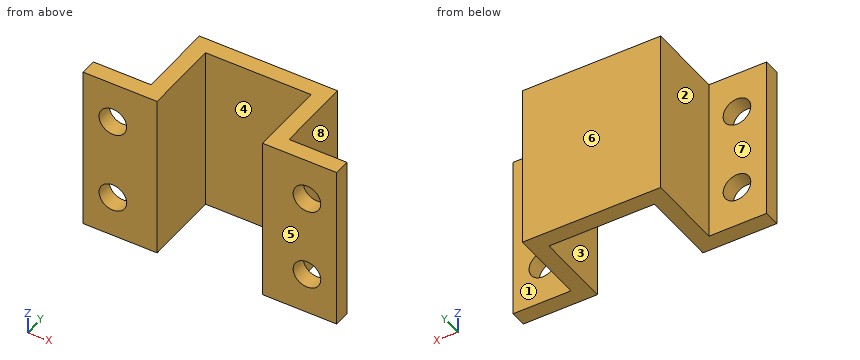
```python
from build123d import *

# Parameters (mm, degrees)
SKETCH1_W             = 9.1
SKETCH1_H             = 20.4
SKETCH1_R             = 1.7
BOSS_EXTRUDE1_DEPTH   = 2
BOSS_EXTRUDE1_2_DEPTH = 2
SKETCH2_W             = 2
SKETCH2_H             = 20.4
BOSS_EXTRUDE2_DEPTH   = 9.49
SKETCH3_W             = 17
SKETCH3_H             = 20.4
BOSS_EXTRUDE3_DEPTH   = 2


with BuildPart() as part:
    # Sketch1 → Boss-Extrude1 (new body)
    with BuildSketch(Plane(origin=(0, 0, 0), x_dir=(1, 0, 0), z_dir=(0, 1, 0))):
        with Locations((-11.05, 0)):
            Rectangle(SKETCH1_W, SKETCH1_H)
        with Locations(Location((-11.95, -5.1, 0), (0, 0, 270))):
            Circle(SKETCH1_R, mode=Mode.SUBTRACT)
        with Locations(Location((-11.95, 5.1, 0), (0, 0, 270))):
            Circle(SKETCH1_R, mode=Mode.SUBTRACT)
    extrude(amount=BOSS_EXTRUDE1_DEPTH)



with BuildPart() as body_2:
    # Sketch1 → Boss-Extrude1 2 (new body)
    with BuildSketch(Plane(origin=(0, 0, 0), x_dir=(1, 0, 0), z_dir=(0, 1, 0))):
        with Locations((11.05, 0)):
            Rectangle(SKETCH1_W, SKETCH1_H)
        with Locations(Location((11.95, -5.1, 0), (0, 0, 270))):
            Circle(SKETCH1_R, mode=Mode.SUBTRACT)
        with Locations(Location((11.95, 5.1, 0), (0, 0, 270))):
            Circle(SKETCH1_R, mode=Mode.SUBTRACT)
    extrude(amount=BOSS_EXTRUDE1_2_DEPTH)


with BuildPart() as part_1:
    add(part.part)

    add(body_2.part)  # Boss-Extrude2 merges body 2
    # Sketch2 → Boss-Extrude2 (add)
    with BuildSketch(Plane(origin=(0, 0, 0), x_dir=(1, 0, 0), z_dir=(0, 1, 0))):
        with Locations((-7.5, 0)):
            Rectangle(SKETCH2_W, SKETCH2_H)
        with Locations((7.5, 0)):
            Rectangle(SKETCH2_W, SKETCH2_H)
    extrude(amount=BOSS_EXTRUDE2_DEPTH)

    # Sketch3 → Boss-Extrude3 (add)
    with BuildSketch(Plane(origin=(0, 9.49, 0), x_dir=(1, 0, 0), z_dir=(0, 1, 0))):
        Rectangle(SKETCH3_W, SKETCH3_H)
    extrude(amount=BOSS_EXTRUDE3_DEPTH)


solid = part_1.part
```
Input: part model. Units: mm. Frame: model coordinates. Face numbers are marked on the shaded views. A direction names the side the tool comes from. Coordinates: 2 decimals unless noted, no trailing zeros. Loops run counter-clockwise (first coordinate to the right, second up) from the corner with the lowest first, then second, coordinate; pieces in that order, holes last. Notation, with made-up numbers: (-15, 37.5) - (26, 37.5) arc R13 cw to (26, 62.5) - close; hole circle Ø10 at (-30.5, 37). An arc over 180 degrees is marked (long way). Answer in a Markdown table with one row per item.
(1) Cut plane B-B on y = 8. Output: boundary loops of the cut face in (x, z), plus the area to 3 significant figures.
Model answer:
| item | result |
|---|---|
| outline | (-8.5, -10.2) - (-6.5, -10.2) - (-6.5, 10.2) - (-8.5, 10.2) - close; (6.5, -10.2) - (8.5, -10.2) - (8.5, 10.2) - (6.5, 10.2) - close |
| area | 81.6 mm² |
(2) Cut plane C-C on x = 11.95. Output: boundary loops of the cut face in (y, z), plus the area to 3 significant figures.
Model answer:
| item | result |
|---|---|
| outline | (0, -10.2) - (2, -10.2) - (2, -6.8) - (0, -6.8) - close; (0, -3.4) - (2, -3.4) - (2, 3.4) - (0, 3.4) - close; (0, 6.8) - (2, 6.8) - (2, 10.2) - (0, 10.2) - close |
| area | 27.2 mm² |
(3) Cut plane D-D on z = -2.5. Output: boundary loops of the cut face in (x, y).
Model answer:
| item | result |
|---|---|
| outline | (-15.6, 0) - (-6.5, 0) - (-6.5, 9.49) - (6.5, 9.49) - (6.5, 0) - (15.6, 0) - (15.6, 2) - (8.5, 2) - (8.5, 11.49) - (-8.5, 11.49) - (-8.5, 2) - (-15.6, 2) - close |
(4) Pin query (flat end, axial travel): P1, Ø3, axis at y = 6.5, z = -5, coming from the -X side; P2, Ø4, axis at x = 1.5, z = 1.5, coming from the -Y side; P3, Ø5.5, axis at x = -11.95, z = 5.1, coming from the +Y side; P4, Ø2.5, axis at x = 11.95, z = 5.1, coming from the +Y side. Return the tip coordinate at first contact, or that it passes through.
Model answer:
| item | result |
|---|---|
| P1 | stops at x = -8.5 |
| P2 | stops at y = 9.49 |
| P3 | stops at y = 2 |
| P4 | passes through |
(5) Material intervals for L1, parallel to X at y = 1.2, z = -5.1; L2, parallel to X at y = 6.5, z = 4; L3, parallel to X at y = 0.75, z = 3.25, sorted ascending. Write a range as from..to.
Model answer:
| item | result |
|---|---|
| L1 | x = -15.6..-13.65, -10.25..-6.5, 6.5..10.25, 13.65..15.6 |
| L2 | x = -8.5..-6.5, 6.5..8.5 |
| L3 | x = -15.6..-6.5, 6.5..15.6 |
(6) Mould query, pull axis X, two halves, no side actions, for the marked faces 1, 2 and 3. Classes: pulls with the +X half, pulls with the -X half, needs draft (parallel to the pull), parting line crosses it, or undercut.
Model answer:
| item | result |
|---|---|
| face 1 | needs draft |
| face 2 | pulls with the -X half |
| face 3 | undercut |
(7) Set-up query: the marked faces 4, 5, 6, 7 and 8. Return all of +Z, -Z, +X, -X, +Y, -Y with unobstructed straight access to the full face (end or side cutting, diameter ignored); none if empty.
Model answer:
| item | result |
|---|---|
| face 4 | +Z, -Z, -Y |
| face 5 | +Z, -Z, +X, -X, -Y |
| face 6 | +Z, -Z, +X, -X, +Y |
| face 7 | +Z, -Z, -X, +Y |
| face 8 | +Z, -Z, +X, +Y |
(8) Cut plane A-A on y = 1.25. Output: boundary loops of the cut face in (x, z).
Model answer:
| item | result |
|---|---|
| outline | (-15.6, -10.2) - (-6.5, -10.2) - (-6.5, 10.2) - (-15.6, 10.2) - close; (6.5, -10.2) - (15.6, -10.2) - (15.6, 10.2) - (6.5, 10.2) - close; hole circle Ø3.4 at (-11.95, -5.1); hole circle Ø3.4 at (-11.95, 5.1); hole circle Ø3.4 at (11.95, -5.1); hole circle Ø3.4 at (11.95, 5.1) |
